Read the model definition and answer for the solid it produces. Units are mm, in the model's axes. Face numbers are marked on the shaded views. A direction names the side the tool comes from. Coordinates: 2 decimals unless noted, no trailing zeros. Write each loop counter-clockwise with the first axis right and the second up, starting at its lowest first coordinate (ties: lowest second). Pieces come first, ordered by that corner, then holes. Notation, with made-up numbers: (24.25, -11.75) -> (48.25, -11.75) arc R14 cw to (48.25, -2.75) -> close; hole circle Ø11 at (-25.5, 86). An arc over 180 degrees is marked (long way). Use CSV: the item, a comma, the result in double quotes.
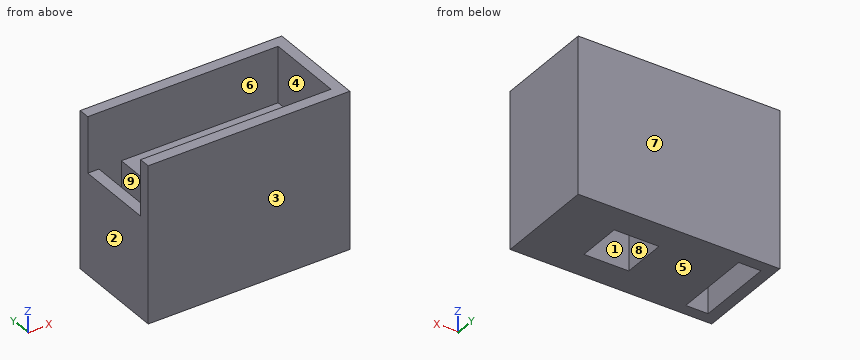
from build123d import *

# Parameters (mm, degrees)
F0_W     = 18
F0_H     = 9
F1_DEPTH = 13
F2_W     = 17
F2_H     = 7
F3_DEPTH = 4
F4_W     = 4
F4_H     = 4
F5_DEPTH = 6
F4_W_2   = 2
F4_H_2   = 7
F6_DEPTH = 9
F8_DEPTH = 1


with BuildPart() as f1:
    # F0 (on Top) → F1 (new body)
    with BuildSketch(Plane.XY):
        Rectangle(F0_W, F0_H)
    extrude(amount=F1_DEPTH)

    # F2 (on face) → F3 (cut)
    with BuildSketch(Plane.XY.offset(13)):
        with Locations((-0.5, 0)):
            Rectangle(F2_W, F2_H)
    extrude(amount=-F3_DEPTH, mode=Mode.SUBTRACT)

    # F4 (on face) → F5 (cut)
    with BuildSketch(Plane(origin=(0, 0, 0), x_dir=(1, 0, 0), z_dir=(0, 0, -1))):
        with Locations((2.1, 0)):
            Rectangle(F4_W, F4_H)
    extrude(amount=-F5_DEPTH, mode=Mode.SUBTRACT)

    # F4 (on face) → F6 (cut)
    with BuildSketch(Plane(origin=(0, 0, 0), x_dir=(1, 0, 0), z_dir=(0, 0, -1))):
        with Locations((-7, 0)):
            Rectangle(F4_W_2, F4_H_2)
    extrude(amount=-F6_DEPTH, mode=Mode.SUBTRACT)

    # F7 (on face) → F8 (join)
    with BuildSketch(Plane.XY.offset(13)):
        Polygon((9, 4.5), (-9, 4.5), (-9, 3.5), (8, 3.5), (8, -3.5), (-9, -3.5), (-9, -4.5), (9, -4.5), align=None)
    extrude(amount=F8_DEPTH)


solid = f1.part
1. For a pull along Y with two mould halves and no side action, classify the marked faces 1, 2, 3 and 4 as pulls with the +Y half, pulls with the -Y half, needs draft (parallel to the pull), parting line crosses it, or undercut.
Solutions:
face 1,"undercut"
face 2,"needs draft"
face 3,"pulls with the -Y half"
face 4,"undercut"
2. Each of these flat-tipped pins is pushed along its axis until it touches: pin 1 Ø1 at (x, y) = (5, 1.5) entering from +Z; pin 2 Ø2.5 at (y, z) = (-0.5, 10.5) entering from -X. Where does it stop, or does it pass through?
Solutions:
pin 1,"stops at z = 9"
pin 2,"stops at x = 8"
3. A cutting plane is placed at D-D (x = 2.75). Give the vertices of the cut face in (y, z), and give its area (3 significant figures).
Solutions:
outline,"(-4.5, 0) -> (-2, 0) -> (-2, 6) -> (2, 6) -> (2, 0) -> (4.5, 0) -> (4.5, 14) -> (3.5, 14) -> (3.5, 9) -> (-3.5, 9) -> (-3.5, 14) -> (-4.5, 14) -> close"
area,"67.0 mm^2"
4. A cutting plane is placed at C-C (z = 1.75). Give the vertices of the cut face in (x, y).
Solutions:
outline,"(-9, -4.5) -> (9, -4.5) -> (9, 4.5) -> (-9, 4.5) -> close; hole (-8, -3.5) -> (-6, -3.5) -> (-6, 3.5) -> (-8, 3.5) -> close; hole (0.1, -2) -> (4.1, -2) -> (4.1, 2) -> (0.1, 2) -> close"
5. Find the intervals of material crossed by line 1 along X through (y, z) = (1.75, 4.5); line 2 along Y through (x, z) = (-5.5, 13); line 3 along X through (y, z) = (1, 8.75), in increasing order.
Solutions:
line 1,"x = -9 to -8, -6 to 0.1, 4.1 to 9"
line 2,"y = -4.5 to -3.5, 3.5 to 4.5"
line 3,"x = -9 to -8, -6 to 9"
6. A cutting plane is placed at B-B (x = -7.5). Give the vertices of the cut face in (y, z).
Solutions:
outline,"(-4.5, 0) -> (-3.5, 0) -> (-3.5, 14) -> (-4.5, 14) -> close; (3.5, 0) -> (4.5, 0) -> (4.5, 14) -> (3.5, 14) -> close"
7. A tool of negligible diameter and unlimited length cuts with its end or side. For the marked faces 5, 6, 7, 8 and 9, from which of +Z, -Z, +X, -X, +Y, -Y can it reach the whole face along a straight path? Write none if from no direction.
Solutions:
face 5,"-Z, +X, -X, +Y, -Y"
face 6,"+Z"
face 7,"+Z, -Z, +X, -X, +Y"
face 8,"-Z"
face 9,"+Z, -Z"
8. A cutting plane is placed at A-A (y = -1.5). Give the vertices of the cut face in (x, z).
Solutions:
outline,"(-9, 0) -> (-8, 0) -> (-8, 9) -> (-9, 9) -> close; (-6, 0) -> (0.1, 0) -> (0.1, 6) -> (4.1, 6) -> (4.1, 0) -> (9, 0) -> (9, 14) -> (8, 14) -> (8, 9) -> (-6, 9) -> close"
